```python
from build123d import *

# Parameters (mm, degrees)
F1_DEPTH = 25.4
F3_DEPTH = 127
F4_R     = 254
F5_DEPTH = 152.4
F6_R     = 241.3
F7_DEPTH = 152.4


with BuildPart() as f1:
    # F0 (on Top) → F1 (new body)
    with BuildSketch(Plane.XY):
        with BuildLine():
            Line((-355.6, 139.1030316258), (-355.6, -318.0850094258))
            ThreePointArc((-355.6, -318.0850094258), (0, -288.925), (355.6, -318.0850094258))
            Line((355.6, -318.0850094258), (355.6, 139.1030316258))
            Line((355.6, 139.1030316258), (101.6, 285.75))
            Line((101.6, 285.75), (-101.6, 285.75))
            Line((-101.6, 285.75), (-355.6, 139.1030316258))
        make_face()
    extrude(amount=F1_DEPTH)

    # F2 (on face) → F3 (join)
    with BuildSketch(Plane.XY.offset(25.4)):
        with BuildLine():
            Line((-209.8065405207, 223.2769247023), (-226.8863032655, 213.4159190839))
            Line((-226.8863032655, 213.4159190839), (-60.1941220043, 46.7237378227))
            ThreePointArc((-60.1941220043, 46.7237378227), (-53.8815367264, 53.8815367264), (-46.7237378227, 60.1941220043))
            Line((-46.7237378227, 60.1941220043), (-209.8065405207, 223.2769247023))
        make_face()
        with BuildLine():
            Line((-60.1941220043, -46.7237378227), (-327.0327279417, -313.5623437601))
            ThreePointArc((-327.0327279417, -313.5623437601), (-311.302932669, -311.2373508984), (-295.5566184449, -309.0270026265))
            Line((-295.5566184449, -309.0270026265), (-46.7237378227, -60.1941220043))
            ThreePointArc((-46.7237378227, -60.1941220043), (-53.8815367264, -53.8815367264), (-60.1941220043, -46.7237378227))
        make_face()
        with BuildLine():
            Line((-75.6023437137, 9.525), (-355.6, 9.525))
            Line((-355.6, 9.525), (-355.6, -9.525))
            Line((-355.6, -9.525), (-75.6023437137, -9.525))
            ThreePointArc((-75.6023437137, -9.525), (-76.2, 0), (-75.6023437137, 9.525))
        make_face()
        with BuildLine():
            Line((226.8863032655, 213.4159190839), (209.8065405207, 223.2769247023))
            Line((209.8065405207, 223.2769247023), (46.7237378227, 60.1941220043))
            ThreePointArc((46.7237378227, 60.1941220043), (53.8815367264, 53.8815367264), (60.1941220043, 46.7237378227))
            Line((60.1941220043, 46.7237378227), (226.8863032655, 213.4159190839))
        make_face()
        with BuildLine():
            Line((355.6, -9.525), (355.6, 9.525))
            Line((355.6, 9.525), (75.6023437137, 9.525))
            ThreePointArc((75.6023437137, 9.525), (76.2, 0), (75.6023437137, -9.525))
            Line((75.6023437137, -9.525), (355.6, -9.525))
        make_face()
        with BuildLine():
            Line((46.7237378227, -60.1941220043), (295.5566184449, -309.0270026265))
            ThreePointArc((295.5566184449, -309.0270026265), (311.302932669, -311.2373508984), (327.0327279417, -313.5623437601))
            Line((327.0327279417, -313.5623437601), (60.1941220043, -46.7237378227))
            ThreePointArc((60.1941220043, -46.7237378227), (53.8815367264, -53.8815367264), (46.7237378227, -60.1941220043))
        make_face()
        with BuildLine():
            Line((-9.525, -75.6023437137), (-9.525, -288.9457819171))
            Line((-9.525, -288.9457819171), (9.525, -288.9457819171))
            Line((9.525, -288.9457819171), (9.525, -75.6023437137))
            ThreePointArc((9.525, -75.6023437137), (0, -76.2), (-9.525, -75.6023437137))
        make_face()
    extrude(amount=F3_DEPTH)

    # F4 (on face) → F5 (join, through all)
    with BuildSketch(Plane(origin=(0, 0, 0), x_dir=(1, 0, 0), z_dir=(0, 0, -1))):
        Circle(F4_R)
    extrude(amount=-F5_DEPTH)

    # F6 (on face) → F7 (cut, through all)
    with BuildSketch(Plane(origin=(0, 0, 0), x_dir=(1, 0, 0), z_dir=(0, 0, -1))):
        Circle(F6_R)
    extrude(amount=-F7_DEPTH, mode=Mode.SUBTRACT)


solid = f1.part
```
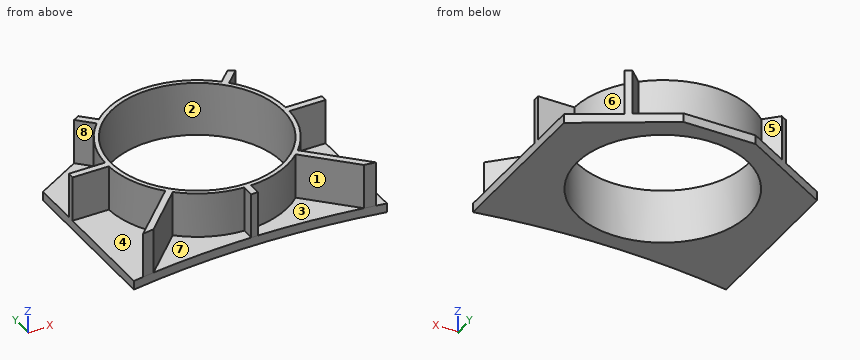
Build history of the part. All positions in model axes, mm. Face numbers are marked on the shaded views. A direction names the side the tool comes from. Give positions to 0.01 mm unless a question says otherwise; leave off trailing zeros. Loops run counter-clockwise (first coordinate to the right, second up) from the corner with the lowest first, then second, coordinate; pieces in that order, holes last. Notation, with made-up numbers: (-14, -39) -> (26, -39) arc R8 cw to (26, -27) -> close; hole circle Ø9 at (-5.5, 63). An arc over 180 degrees is marked (long way). One line per question, with ' | ' between items. Start each with the question number.
1) Cut at D-D (y = -74). Give the cut face in (x, z).
2) Two-plate mould, pull along Y, no slides. Class the marked faces 1, 2, 3 and 4: released by +Y, released by -Y, zero draft, split by the parting line, or undercut.
3) Cut at A-A (x = 0). Give the cut face in (y, z) (3 decimals).
4) Pin check, flat tips, straight feed: pin 1 (3 mm diameter, centred on y = -219, z = 41, fed in from -X); pin 2 (17.5 mm diameter, centred on y = -267, z = 59, fed in from -X); pin 3 (1 mm diameter, centred on x = 55.5, z = 39, fed in from -Y). Stop position of each tip, or through.
5) Cut at B-B (y = 0). Give the cut face in (x, z), plus the area to 3 significant figures.
6) 3-axis set-ups, long thin cutter, end or side, ignore diameter. For the marked faces 5, 6, 7 and 8: which of +Z, -Z, +X, -X, +Y, -Y reach the whole face in a straight line?
7) Probe L1, parallel to X at y = 0, z = 87; L2, parallel to Y at x = 0, z = 105; L3, parallel to Y at x = -192, z = 34. List the from-to ranges inside material, lowest first.
8) Cut at C-C (x = 305). Give the cut face in (y, z) (3 decimals).
Return value:
1) outline: (-355.6, 0) -> (-229.67, 0) -> (-229.67, 152.4) -> (-242.98, 152.4) -> (-242.98, 25.4) -> (-355.6, 25.4) -> close; (229.67, 0) -> (355.6, 0) -> (355.6, 25.4) -> (242.98, 25.4) -> (242.98, 152.4) -> (229.67, 152.4) -> close
2) face 1: released by -Y | face 2: undercut | face 3: zero draft | face 4: undercut
3) outline: (-288.946, 25.4) -> (-288.925, 25.4) -> (-288.925, 0) -> (-241.3, 0) -> (-241.3, 152.4) -> (-288.946, 152.4) -> close; (241.3, 0) -> (285.75, 0) -> (285.75, 25.4) -> (254, 25.4) -> (254, 152.4) -> (241.3, 152.4) -> close
4) pin 1: x = -233.97 | pin 2: x = -289.22 | pin 3: y = -247.97
5) outline: (-355.6, 0) -> (-241.3, 0) -> (-241.3, 152.4) -> (-355.6, 152.4) -> close; (241.3, 0) -> (355.6, 0) -> (355.6, 152.4) -> (241.3, 152.4) -> close | area: 34,800 mm^2
6) face 5: +Z, +Y | face 6: +Z, +X | face 7: +Z, -Y | face 8: +Z, -X
7) L1: -355.6 to -241.3, 241.3 to 355.6 | L2: -288.95 to -241.3, 241.3 to 254 | L3: -205.47 to -178.53, -166.29 to -146.16, 146.16 to 166.29, 178.53 to 205.47
8) outline: (-310.339, 0) -> (168.317, 0) -> (168.317, 25.4) -> (9.525, 25.4) -> (9.525, 152.4) -> (-9.525, 152.4) -> (-9.525, 25.4) -> (-291.53, 25.4) -> (-291.53, 152.4) -> (-310.339, 152.4) -> close
